Input: part model. Units: mm. Frame: model coordinates. A direction names the side the tool comes from. Coordinates: 2 decimals unless noted, no trailing zeros. Loops run counter-clockwise (first coordinate to the right, second up) from the corner with the lowest first, then second, coordinate; pieces in that order, holes last. Notation, with made-up numbers: (-31.75, 42) - (-14.75, 42) arc R26 ccw to (-14.75, 68) - close; hole circle Ø9 at (-26, -9.75). An arc over 180 degrees is marked (long way). Answer as CSV lines item,"result". Start each with the question number.
```python
from build123d import *

# Parameters (mm, degrees)
F0_W     = 21
F0_H     = 4
F5_DEPTH = 1.5
F6_SIZE  = 0.3


with BuildPart() as f2:
    # F0 (on Front) → F2 (revolve)
    with BuildSketch(Plane.XZ):
        Polygon((0, 4), (0, 0), (84, 0), (84, 7), (48, 7), (48, 5), (46.5, 5), (45, 5), (23, 5), (20, 5), (20, 2.5), (18, 2.5), (18, 4), align=None)
        Polygon((84, 7), (84, 0), (99, 0), (99, 4), (99, 5), (89, 5), (85, 9), (84, 9), align=None)
        with Locations((109.5, 2)):
            Rectangle(F0_W, F0_H)
    revolve(axis=Axis((63.735422, 0, 0), (1, 0, 0)))

    # F4 (on offset) → F5 (cut, through all)
    with BuildSketch(Plane.XY.offset(3.5)):
        with BuildLine():
            Line((45.000072, 1.5), (23.000072, 1.5))
            ThreePointArc((23.000072, 1.5), (21.939412, 1.06066), (21.500072, 0))
            ThreePointArc((21.500072, 0), (21.939412, -1.06066), (23.000072, -1.5))
            Line((23.000072, -1.5), (45.000072, -1.5))
            ThreePointArc((45.000072, -1.5), (46.060732, -1.06066), (46.500072, 0))
            ThreePointArc((46.500072, 0), (46.060732, 1.06066), (45.000072, 1.5))
        make_face()
    extrude(amount=F5_DEPTH, mode=Mode.SUBTRACT)

    # F6
    f6_edges = [f2.edges().sort_by_distance(p)[0] for p in [
        (120, 0, -4),
        (99, 0, -5),
        (48, 0, -7),
        (20, 0, -5),
        (0, 0, -4),
    ]]
    chamfer(f6_edges, length=F6_SIZE)


solid = f2.part
```
Item 1: Contact query for flat-ended pins moving along their axis: P1, Ø6, axis at y = -4, z = -4, coming from the -X side; P2, Ø4, axis at x = 44.5, y = -6.5, coming from the +Z side; P3, Ø3.5, axis at x = 31.5, y = -0.5, coming from the +Z side; P4, Ø3, axis at x = 97.5, y = 5, coming from the +Z side. Output: stop coordinate, or through.
Item 2: Draft query along X for faces 1 (the cylindrical face through (65.9, 2.681, 6.466)), 2 (the flat face through (18, -2, -2)), 3 (the flat face through (120, 0, 0)). Return one class per face: pulls with the +X half, pulls with the -X half, needs draft (parallel to the pull), parting line crosses it, or undercut.
Item 3: Material intervals for probe 1 along X at (y, z) = (-3, -1); probe 2 along X at (y, z) = (-0.5, -4); probe 3 along Y at (x, z) = (50, 0.25), sorted ascending.
Item 4: Section query A-A, the plane x = 15.5. Output: boundary loops of the cut face in (y, z), and give its area (3 significant figures).
Item 5: Set-up query: faces 4 (the flat face through (84, 7.3, 0)), 5 (the cylindrical face through (93.78, 4.88, -1.08)), 6 (the cylindrical face through (18.99, 2.44, -0.54)), 7 (the cylindrical face through (84.493, -8.923, -1.172)). Return all of +Z, -Z, +X, -X, +Y, -Y with unobstructed straight access to the full face (end or side cutting, diameter ignored); none if empty.
Response values:
1,P1,"stops at x = 0"
1,P2,"stops at z = 2.18"
1,P3,"stops at z = 4.77"
1,P4,"stops at z = 3.57"
2,face 1,"needs draft"
2,face 2,"undercut"
2,face 3,"pulls with the +X half"
3,probe 1,"x = 0 to 18, 20 to 120"
3,probe 2,"x = 20 to 99"
3,probe 3,"y = -7 to 7"
4,outline,"circle Ø8 at (0, 0)"
4,area,"50.3 mm²"
5,face 4,"-X"
5,face 5,"+X"
5,face 6,"none"
5,face 7,"+X, -X"
